Here's how the part is built. I have some questions about the finished solid (model axes, mm). Face numbers are marked on the shaded views. A direction names the side the tool comes from. Coordinates: 2 decimals unless noted, no trailing zeros. Order: outer loops, then holes, each group sorted by start corner. A loop starts at its lowest first (then second) coordinate and runs counter-clockwise, first axis right, second up. Notation, with made-up numbers: (26, -30.75) - (39, -30.75) arc R19 cw to (39, 4.25) - close; hole circle Ø11 at (38, 41.25). An arc over 180 degrees is marked (long way). Answer as CSV lines item,"result". Start each with the question number.
Q1. For the marked faces 1 and 2, which set-ups out of +Z, -Z, +X, -X, +Y, -Y let a thin tool reach every point of the face, with its end or its side?
Q2. Suppose I cut it at C-C (z = -3). Count the separate pieces of the cut face and the enclosed holes in it, then the cut area to 3 significant figures.
Q3. I need wall thicknesses on line 1 (X direction, y = 74.5, z = 5); line 2 (Y direction, x = -8, z = 2.25); line 3 (X direction, y = 104, z = -1.25). Which ranges of each line are inside material? Lowest first, please.
Q4. For pin 1 Ø8 at (y, z) = (20.5, 3.5) entering from +X (3 decimals); pin 2 Ø8 at (x, z) = (14.5, 0.5) entering from -Y; pin 3 Ø5 at (y, z) = (28.5, 2) entering from -X, each with a flat end and sliding along its axis, tell me the tip position at first contact or that it passes through.
Q5. Suppose I cut it at D-D (x = 48). Please give me the cut outline in (y, z).
Q6. Suppose I cut it at B-B (y = 66.5). Please give me the cut outline in (x, z), then the cut area to 3 significant figures.
Q7. Thinking about a two-plate mould opening in X: for the marked faces 3, 4 and 5, which applies, released by +X, released by -X, zero draft, split by the parting line, or undercut?
Q8. Suppose I cut it at A-A (x = -8). Please give me the cut outline in (y, z), then the cut area to 3 significant figures.
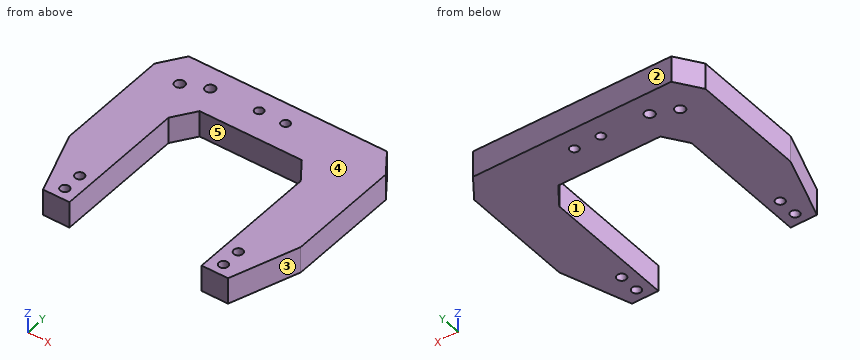
from build123d import *

# Parameters (mm, degrees)
DODANIE_WYCI_GNI_CIE1_DEPTH                       = 8
POG_BIENIE_WALCOWE_POD_M5_RUB_Z_BEM_W_D           = 5.3
POG_BIENIE_WALCOWE_POD_M5_RUB_Z_BEM_W_DEPTH       = 60
POG_BIENIE_WALCOWE_POD_M5_RUB_Z_BEM_W_CBORE_D     = 10
POG_BIENIE_WALCOWE_POD_M5_RUB_Z_BEM_W_CBORE_DEPTH = 2
POG_BIENIE_WALCOWE_POD_M5_RUB_Z_BEM_W_TIP         = 1.59228064
POG_BIENIE_WALCOWE_POD_M5_RUB_Z_B_2_A_COUNT       = 2
POG_BIENIE_WALCOWE_POD_M5_RUB_Z_B_2_A_PITCH       = 12
OTWORY_USTALAJ_CE_6_0MM1_D                        = 6
OTWORY_USTALAJ_CE_6_0MM1_DEPTH                    = 32
OTWORY_USTALAJ_CE_6_0MM1_TIP                      = 1.802581857


with BuildPart() as part:
    # Szkic1 → Dodanie-wyciągnięcie1 (new, symmetric)
    with BuildSketch(Plane.XY):
        Polygon((0, 93), (0, 123), (60, 123), (70, 108.718519933), (70, 40), (56, 0), (40, 0), (40, 80), (30.897302003, 93), align=None)
    dodanie_wyci_gni_cie1 = extrude(amount=DODANIE_WYCI_GNI_CIE1_DEPTH, both=True)

    # Lustro1: Dodanie-wyciągnięcie1 across plane
    add(dodanie_wyci_gni_cie1.mirror(Plane(origin=(0, 93, 8), x_dir=(0, 0, 1), z_dir=(1, 0, 0))))

    # Pog_bienie walcowe pod M5 _rub_ z _bem w
    with Locations(Plane(origin=(156.349537134, 156, 18.427358502), x_dir=(1, 0, 0), z_dir=(0, 0, 1))):
        with Locations((-164.349537134, -45.5), (-148.349537134, -45.5)):
            CounterBoreHole(POG_BIENIE_WALCOWE_POD_M5_RUB_Z_BEM_W_D / 2, POG_BIENIE_WALCOWE_POD_M5_RUB_Z_BEM_W_CBORE_D / 2, POG_BIENIE_WALCOWE_POD_M5_RUB_Z_BEM_W_CBORE_DEPTH, depth=POG_BIENIE_WALCOWE_POD_M5_RUB_Z_BEM_W_DEPTH)
            with Locations((0, 0, -(POG_BIENIE_WALCOWE_POD_M5_RUB_Z_BEM_W_DEPTH + POG_BIENIE_WALCOWE_POD_M5_RUB_Z_BEM_W_TIP / 2))):  # 118° drill point
                Cone(0, POG_BIENIE_WALCOWE_POD_M5_RUB_Z_BEM_W_D / 2, POG_BIENIE_WALCOWE_POD_M5_RUB_Z_BEM_W_TIP, mode=Mode.SUBTRACT)

    # Szkic9 → Pog_bienie walcowe pod M5 _rub_ z _b 2 (revolve, cut)
    with BuildSketch(Plane(origin=(-48, 7, -22), x_dir=(0, 1, 0), z_dir=(1, 0, 0))):
        Polygon((0, 0), (0, 45.652366702), (2.75, 44), (2.75, 5), (5, 5), (5, 0), align=None)
    pog_bienie_walcowe_pod_m5_rub_z_b_2 = revolve(axis=Axis((-48, 7, -28.35), (0, 0, 1)), mode=Mode.SUBTRACT)

    # Pog_bienie walcowe pod M5 _rub_ z _b 2 a: Pog_bienie walcowe pod M5 _rub_ z _b 2 ×2
    with Locations(*[(0, i * POG_BIENIE_WALCOWE_POD_M5_RUB_Z_B_2_A_PITCH, 0) for i in range(1, POG_BIENIE_WALCOWE_POD_M5_RUB_Z_B_2_A_COUNT)]):
        add(pog_bienie_walcowe_pod_m5_rub_z_b_2, mode=Mode.SUBTRACT)

    # Lustro2: Pog_bienie walcowe pod M5 _rub_ z _b 2 across plane
    add(pog_bienie_walcowe_pod_m5_rub_z_b_2.mirror(Plane(origin=(0, 0, 0), x_dir=(0, 0, 1), z_dir=(1, 0, 0))), mode=Mode.SUBTRACT)

    # Lustro2 copy 1 sketch → Lustro2 copy 1 (revolve, cut)
    with BuildSketch(Plane(origin=(48, 19, -22), x_dir=(0, 1, 0), z_dir=(-1, 0, 0))):
        Polygon((0, 0), (0, -45.652366702), (2.75, -44), (2.75, -5), (5, -5), (5, 0), align=None)
    revolve(axis=Axis((48, 19, -28.35), (0, 0, -1)), mode=Mode.SUBTRACT)

    # Otwory ustalające Ø6.0mm1
    with Locations(Plane(origin=(156.349537134, 156, 8), x_dir=(1, 0, 0), z_dir=(0, 0, 1))):
        with Locations((-193.349537133, -46.25), (-207.349537133, -52.25)):
            Hole(OTWORY_USTALAJ_CE_6_0MM1_D / 2, depth=OTWORY_USTALAJ_CE_6_0MM1_DEPTH)
            with Locations((0, 0, -(OTWORY_USTALAJ_CE_6_0MM1_DEPTH + OTWORY_USTALAJ_CE_6_0MM1_TIP / 2))):  # 118° drill point
                Cone(0, OTWORY_USTALAJ_CE_6_0MM1_D / 2, OTWORY_USTALAJ_CE_6_0MM1_TIP, mode=Mode.SUBTRACT)


solid = part.part
Here are the results:
1,face 1,"+Z, -Z, -Y"
1,face 2,"+Z, -Z, +X, -X, +Y"
2,separate pieces,"1"
2,enclosed holes,"8"
2,area,"9,000 mm²"
3,line 1,"x = -70 to -40, 40 to 70"
3,line 2,"y = 93 to 107.85, 113.15 to 123"
3,line 3,"x = -70 to -53.99, -48.01 to 70"
4,pin 1,"stops at x = 64.575"
4,pin 2,"stops at y = 93"
4,pin 3,"stops at x = -66.85"
5,outline,"(0, -8) - (4.25, -8) - (4.25, 8) - (0, 8) - close; (9.75, -8) - (16.25, -8) - (16.25, 8) - (9.75, 8) - close; (21.75, -8) - (123, -8) - (123, 8) - (21.75, 8) - close"
6,outline,"(-70, -8) - (-40, -8) - (-40, 8) - (-70, 8) - close; (40, -8) - (70, -8) - (70, 8) - (40, 8) - close"
6,area,"960 mm²"
7,face 3,"released by +X"
7,face 4,"zero draft"
7,face 5,"undercut"
8,outline,"(93, -8) - (107.85, -8) - (107.85, 8) - (93, 8) - close; (113.15, -8) - (123, -8) - (123, 8) - (113.15, 8) - close"
8,area,"395 mm²"
